from build123d import *

# Parameters (mm, degrees)
SKETCH1_W               = 13.8
SKETCH1_H               = 8.8
BOSS_EXTRUDE1_DEPTH     = 3
SKETCH2_W               = 2
SKETCH2_H               = 35
BOSS_EXTRUDE2_DEPTH     = 3
SKETCH3_W               = 1.2
SKETCH3_H               = 6
BOSS_EXTRUDE3_DEPTH     = 7
FILLET3_R               = 10
SKETCH5_W               = 15
SKETCH5_H               = 13.8
BOSS_EXTRUDE4_DEPTH     = 4
SKETCH6_R               = 1.5
CUT_EXTRUDE4_DEPTH      = 38.968539608
BOSS_EXTRUDE5_DEPTH     = 2
CHAMFER2_SIZE           = 3
BOSS_EXTRUDE7_DEPTH     = 1.2
SKETCH12_W              = 15
SKETCH12_H              = 4
BOSS_EXTRUDE8_DEPTH     = 3
SKETCH13_W              = 15
SKETCH13_H              = 4
BOSS_EXTRUDE9_DEPTH     = 3
CUT_EXTRUDE7_DEPTH      = 43.28486727
CUT_EXTRUDE7_DEPTH_BACK = 43.28486727
CUT_EXTRUDE8_DEPTH      = 43.28486727
CUT_EXTRUDE8_DEPTH_BACK = 43.28486727
SKETCH15_W              = 0.807911756
SKETCH15_H              = 0.64
CUT_EXTRUDE9_DEPTH      = 41.244591358
CUT_EXTRUDE9_DEPTH_BACK = 41.244591358
SKETCH16_W              = 0.64
SKETCH16_H              = 0.6
CHAMFER3_SIZE           = 1
SKETCH18_W              = 20.701942652
SKETCH18_H              = 41.728044518
CUT_EXTRUDE10_DEPTH     = 36
SKETCH19_W              = 11.097134513
SKETCH19_H              = 20.928514419
CUT_EXTRUDE11_DEPTH     = 3.5


# Some blends are built 0.0001 mm under size
with BuildPart() as part:
    # Sketch1 → Boss-Extrude1 (new body)
    with BuildSketch(Plane(origin=(0, 0, 0), x_dir=(0, 0, -1), z_dir=(1, 0, 0))):
        Rectangle(SKETCH1_W, SKETCH1_H)
    extrude(amount=BOSS_EXTRUDE1_DEPTH)

    # Sketch2 → Boss-Extrude2 (add)
    with BuildSketch(Plane(origin=(3, 0, 0), x_dir=(0, 0, -1), z_dir=(1, 0, 0))):
        with Locations((0, -13.1)):
            Rectangle(SKETCH2_W, SKETCH2_H)
    extrude(amount=BOSS_EXTRUDE2_DEPTH)

    # Sketch3 → Boss-Extrude3 (add)
    with BuildSketch(Plane(origin=(6, 0, 0), x_dir=(0, 0, -1), z_dir=(1, 0, 0))):
        with Locations((0, -27.6)):
            Rectangle(SKETCH3_W, SKETCH3_H)
    extrude(amount=BOSS_EXTRUDE3_DEPTH)

    # Fillet3
    # the kernel refuses this fillet: 10 mm, written as the material it adds along each edge
    with BuildSketch(Plane(origin=(3, -4.4, 1), x_dir=(-1, 0, 0), z_dir=(0, 0, -1))) as fillet3_piece_1:
        with BuildLine():
            CenterArc((10, -7.141428429), FILLET3_R, 134.427004001, 45.572995999)
            Line((0, -7.141428429), (0, 0))
            Line((0, 0), (3, 0))
        make_face()
    extrude(amount=2)

    # Sketch5 → Boss-Extrude4 (add)
    with BuildSketch(Plane(origin=(0, 4.4, 0), x_dir=(1, 0, 0), z_dir=(0, 1, 0))):
        with Locations((-4.5, 0)):
            Rectangle(SKETCH5_W, SKETCH5_H)
    extrude(amount=BOSS_EXTRUDE4_DEPTH)

    # Sketch6 → Cut-Extrude4 (cut, through all)
    with BuildSketch(Plane.XZ.offset(-4.4)):
        with Locations(Location((-6, 3, 0), (0, 0, 270))):
            Circle(SKETCH6_R)
        with Locations(Location((-6, -3, 0), (0, 0, 270))):
            Circle(SKETCH6_R)
    extrude(amount=-CUT_EXTRUDE4_DEPTH, mode=Mode.SUBTRACT)

    # Sketch8 → Boss-Extrude5 (add)
    with BuildSketch(Plane(origin=(0, 0, -1), x_dir=(-1, 0, 0), z_dir=(0, 0, -1))):
        Polygon((-3, -18.758153574), (0, -4.4), (-3, -4.4), align=None)
    extrude(amount=-BOSS_EXTRUDE5_DEPTH)

    # Chamfer2
    chamfer2_edges = [part.edges().sort_by_distance(p)[0] for p in [
        (3, 4.4, 0),
    ]]
    chamfer(chamfer2_edges, length=CHAMFER2_SIZE - 0.0001)  # a hair under: the kernel refuses the full size

    # Sketch11 → Boss-Extrude7 (add)
    with BuildSketch(Plane(origin=(0, 0, -0.6), x_dir=(-1, 0, 0), z_dir=(0, 0, -1))):
        Polygon((-6, -24.6), (-13, -24.6), (-6, 1.742521041), align=None)
    extrude(amount=-BOSS_EXTRUDE7_DEPTH)

    # Sketch12 → Boss-Extrude8 (add)
    with BuildSketch(Plane(origin=(0, 0, -6.9), x_dir=(-1, 0, 0), z_dir=(0, 0, -1))):
        with Locations((4.5, 6.4)):
            Rectangle(SKETCH12_W, SKETCH12_H)
    extrude(amount=BOSS_EXTRUDE8_DEPTH)

    # Sketch13 → Boss-Extrude9 (add)
    with BuildSketch(Plane.XY.offset(6.9)):
        with Locations((-4.5, 6.4)):
            Rectangle(SKETCH13_W, SKETCH13_H)
    extrude(amount=BOSS_EXTRUDE9_DEPTH)

    # Sketch14 → Cut-Extrude7 (cut, two sides: drawn at the far end of the back side and taken through both)
    with BuildSketch(Plane(origin=(0, 8.4, 0), x_dir=(1, 0, 0), z_dir=(0, 1, 0)).offset(-CUT_EXTRUDE7_DEPTH_BACK)):
        with BuildLine():
            Line((-7.5, 7), (-7.5, -7))
            ThreePointArc((-7.5, -7), (-6, -8.5), (-4.5, -7))
            Line((-4.5, -7), (-4.5, 7))
            ThreePointArc((-4.5, 7), (-6, 8.5), (-7.5, 7))
        make_face()
    extrude(amount=CUT_EXTRUDE7_DEPTH + CUT_EXTRUDE7_DEPTH_BACK, mode=Mode.SUBTRACT)

    # Sketch15 → Cut-Extrude8 (cut, two sides: drawn at the far end of the back side and taken through both)
    with BuildSketch(Plane.XZ.offset(30.6).offset(-CUT_EXTRUDE8_DEPTH_BACK)):
        with Locations((12.596044122, 0)):
            Rectangle(SKETCH15_W, SKETCH15_H)
    extrude(amount=CUT_EXTRUDE8_DEPTH + CUT_EXTRUDE8_DEPTH_BACK, mode=Mode.SUBTRACT)

    # Sketch16 → Cut-Extrude9 (cut, two sides: drawn at the far end of the back side and taken through both)
    with BuildSketch(Plane(origin=(12.192088244, 0, 0), x_dir=(0, 0, -1), z_dir=(1, 0, 0)).offset(-CUT_EXTRUDE9_DEPTH_BACK)):
        with Locations((0, -30.3)):
            Rectangle(SKETCH16_W, SKETCH16_H)
    extrude(amount=CUT_EXTRUDE9_DEPTH + CUT_EXTRUDE9_DEPTH_BACK, mode=Mode.SUBTRACT)

    # Chamfer3
    chamfer3_edges = [part.edges().sort_by_distance(p)[0] for p in [
        (12.192088244, -30, 0),
    ]]
    chamfer(chamfer3_edges, length=CHAMFER3_SIZE)

    # Sketch18 → Cut-Extrude10 (cut)
    with BuildSketch(Plane.XY.offset(9.9)):
        with Locations((9.448105839, -12.464022259)):
            Rectangle(SKETCH18_W, SKETCH18_H)
    extrude(amount=-CUT_EXTRUDE10_DEPTH, mode=Mode.SUBTRACT)

    # Sketch19 → Cut-Extrude11 (cut)
    with BuildSketch(Plane.XZ.offset(-4.4)):
        with Locations((-6.451432743, 0.56425721)):
            Rectangle(SKETCH19_W, SKETCH19_H)
    extrude(amount=-CUT_EXTRUDE11_DEPTH, mode=Mode.SUBTRACT)


solid = part.part
Here's how the part is built. I have some questions about the finished solid (model axes, mm). Coordinates: 2 decimals unless noted, no trailing zeros. Order: outer loops, then holes, each group sorted by start corner. A loop starts at its lowest first (then second) coordinate and runs counter-clockwise, first axis right, second up. Notation, with made-up numbers: M 47.25,51 L 100.25,51 A12 cw 100.25,64 Z; hole C 70.5,30 d5. An arc over 180 degrees is marked long. Answer as CSV lines item,"result". Start each with the question number.
1. I need wall thicknesses on line 1 (X direction, y = 8.1, z = 0.75); line 2 (Z direction, x = -6, y = 8.1); line 3 (Z direction, x = -7, y = 8.1). Which ranges of each line are inside material? Lowest first, please. Write a range as [from, to].
2. We'd pull the mould along X, two halves only. Please class faces 1 (the cylindrical face through (-6, 8.1, 8.5)), 2 (the flat face through (-8, 7.9, 0)), 3 (the cylindrical face through (-6, 8.1, -8.5)): released by +X, released by -X, zero draft, split by the parting line, or undercut.
3. I want a section at C-C, the plane y = 8.05. Write out the boundary of the cut face in (x, z).
4. I want a section at A-A, the plane x = -6. Write out the boundary of the cut face in (y, z).
5. I want a section at B-B, the plane z = -0.75. Write out the boundary of the cut face in (x, y), and give its area (3 significant figures).
Recorded:
1,line 1,"x = [-12, -7.5], [-4.5, -0.9]"
1,line 2,"z = [-9.9, -8.5], [8.5, 9.9]"
1,line 3,"z = [-9.9, -8.12], [8.12, 9.9]"
2,face 1,"undercut"
2,face 2,"zero draft"
2,face 3,"undercut"
3,outline,"M -12,-9.9 L -0.9,-9.9 L -0.9,9.9 L -12,9.9 Z; hole M -7.5,-7 A1.5 ccw -4.5,-7 L -4.5,7 A1.5 ccw -7.5,7 Z"
4,outline,"M 7.9,-9.9 L 8.4,-9.9 L 8.4,-8.5 L 7.9,-8.5 Z; M 7.9,8.5 L 8.4,8.5 L 8.4,9.9 L 7.9,9.9 Z"
5,outline,"M -12,7.9 L -7.5,7.9 L -7.5,8.4 L -12,8.4 Z; M -4.5,7.9 L -0.9,7.9 L -0.9,8.4 L -4.5,8.4 Z"
5,area,"4.05 mm2"
